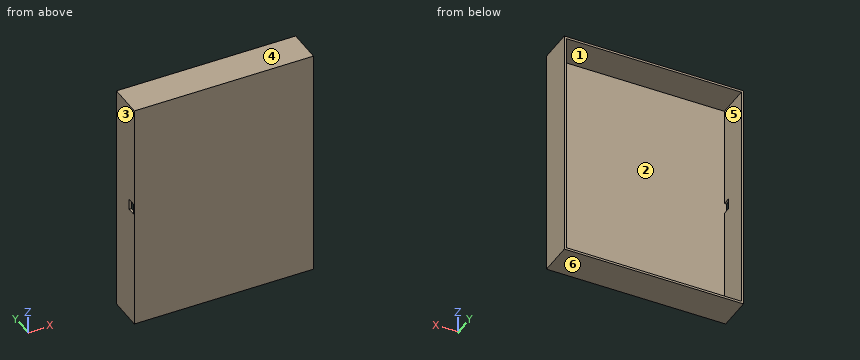
Autodesk Inventor part; units mm, degrees
ref_plane "YZ Plane" through (0, 0, 0) normal (1, 0, 0) x (0, 1, 0)
ref_plane "XZ Plane" through (0, 0, 0) normal (0, 1, 0) x (-1, 0, 0)
ref_plane "XY Plane" through (0, 0, 0) normal (0, 0, 1) x (1, 0, 0)
sketch "Szkic1" plane through (0, 0, 0) normal (0, 1, 0) x (-1, 0, 0)
  line L0 (-165, -215) -> (165, -215)
  line L1 (165, -215) -> (165, 215)
  line L2 (165, 215) -> (-165, 215)
  line L3 (-165, 215) -> (-165, -215)
  line L4 (-165, -215) -> (165, 215) construction
  line L5 (165, -215) -> (-165, 215) construction
  point P0 (0, 0)
  dimension "d0" = 430
  dimension "d1" = 330
extrude "Wyciągnięcie proste1" add sketch "Szkic1" along normal mid plane 3
sketch "Szkic2" plane through (0, 1.5, 0) normal (0, 1, 0) x (1, 0, 0)
  line L0 (161, -211) -> (-161, -211)
  line L1 (-161, -211) -> (-161, 211)
  line L2 (-161, 211) -> (161, 211)
  line L3 (161, 211) -> (161, -211)
  line L4 (161, -211) -> (-161, 211) construction
  line L5 (-161, -211) -> (161, 211) construction
  line L6 (-165, 215) -> (-165, -215)
  line L7 (-165, -215) -> (165, -215)
  line L8 (165, -215) -> (165, 215)
  line L9 (165, 215) -> (-165, 215)
  point P0 (0, 0)
  dimension "d4" = 322
  dimension "d5" = 422
extrude "Wyciągnięcie proste2" add sketch "Szkic2" along normal blind 60
sketch "Szkic4" plane through (-165, -1.5, -215) normal (-1, 0, 0) x (0, 0, 1)
  line L0 (426, 3) -> (4, 3)
  line L1 (220, 3) -> (240, 3)
  line L2 (240, 3) -> (240, 18)
  line L3 (240, 18) -> (220, 18)
  line L4 (220, 18) -> (220, 3)
  line L5 (430, 0) -> (430, 63)
  point P0 (215, 1.5)
  dimension "d13" = 20
  dimension "d14" = 15
  dimension "d15" = 190
extrude "Wyciągnięcie proste4" cut sketch "Szkic4" against normal up to surface (4 mm away)
properties part number "BaseFloor"
Build history of the part. All positions in model axes, mm. Face numbers are marked on the shaded views. A direction names the side the tool comes from. Round coordinates to 2 decimals unless told otherwise and drop trailing zeros. Order: outer loops, then holes, each group sorted by start corner. A loop starts at its lowest first (then second) coordinate and runs counter-clockwise, first axis right, second up. Notation, with made-up numbers: (-23.75, 20.25) -> (15.25, 20.25) arc R5 ccw to (15.25, 27.25) -> close; hole circle Ø4 at (-1, 30). An arc over 180 degrees is marked (long way). Answer in a Markdown table with one row per item.
1) Mould opens along Z. For the marked faces 1, 2, 3 and 4 say: released by +Z, released by -Z, zero draft, split by the parting line, or undercut.
Values:
| item | result |
|---|---|
| face 1 | undercut |
| face 2 | undercut |
| face 3 | zero draft |
| face 4 | released by +Z |
2) Band-saw the part on C-C on x = -40.5. Give the cut face in (y, z).
Values:
| item | result |
|---|---|
| outline | (-1.5, -215) -> (61.5, -215) -> (61.5, -211) -> (1.5, -211) -> (1.5, 211) -> (61.5, 211) -> (61.5, 215) -> (-1.5, 215) -> close |
3) Pin check, flat tip, straight feed: P1, Ø6, axis at x = -62, z = 80.5, coming from the +Y side. Stop position of the tip, or through.
Values:
| item | result |
|---|---|
| P1 | y = 1.5 |
4) Band-saw the part on A-A on z = 14. Give the cut face in (x, y).
Values:
| item | result |
|---|---|
| outline | (-165, -1.5) -> (165, -1.5) -> (165, 61.5) -> (161, 61.5) -> (161, 1.5) -> (-165, 1.5) -> close; (-165, 16.5) -> (-161, 16.5) -> (-161, 61.5) -> (-165, 61.5) -> close |
5) Band-saw the part on B-B on y = 46. Give the cut face in (x, z).
Values:
| item | result |
|---|---|
| outline | (-165, -215) -> (165, -215) -> (165, 215) -> (-165, 215) -> close; hole (-161, -211) -> (161, -211) -> (161, 211) -> (-161, 211) -> close |
6) Band-saw the part on D-D on y = 9.5. Give the cut face in (x, z), and give its area (3 significant figures).
Values:
| item | result |
|---|---|
| outline | (-165, -215) -> (165, -215) -> (165, 215) -> (-165, 215) -> (-165, 25) -> (-161, 25) -> (-161, 211) -> (161, 211) -> (161, -211) -> (-161, -211) -> (-161, 5) -> (-165, 5) -> close |
| area | 5,940 mm2 |
7) Wall check: L1, parallel to X at y = 11, z = 81; L2, parallel to Z at x = 137.5, y = 28.5; L3, parallel to Y at x = -15, z = 38.5. Give the ranges that are in metal, low to high.
Values:
| item | result |
|---|---|
| L1 | -165 to -161, 161 to 165 |
| L2 | -215 to -211, 211 to 215 |
| L3 | -1.5 to 1.5 |
8) Which spindle directions (+Z, -Z, +X, -X, +Y, -Y) get a long thin tool onto all of the face, cutting with end or side? Do the marked faces 5 and 6. Say none if no direction does.
Values:
| item | result |
|---|---|
| face 5 | +Y |
| face 6 | -Z, +X, -X, +Y, -Y |
